```python
from build123d import *

# Parameters (mm, degrees)
F0_W     = 20
F0_H     = 20
F1_DEPTH = 5
F2_R     = 3
F2_R_2   = 1.375
F3_DEPTH = 25
F4_R     = 5
F5_DEPTH = 3.5
F6_R     = 7.5
F7_DEPTH = 1.5


with BuildPart() as f1:
    # F0 (on Top) → F1 (new body)
    with BuildSketch(Plane.XY):
        with Locations((10, 10)):
            Rectangle(F0_W, F0_H)
    extrude(amount=F1_DEPTH)

    # F2 (on face) → F3 (cut)
    with BuildSketch(Plane.XY.offset(5)):
        with Locations((10, 10)):
            Circle(F2_R)
        with Locations((2.5, 17.5)):
            Circle(F2_R_2)
        with Locations((17.5, 17.5)):
            Circle(F2_R_2)
        with Locations((17.5, 2.5)):
            Circle(F2_R_2)
        with Locations((2.5, 2.5)):
            Circle(F2_R_2)
    extrude(amount=-F3_DEPTH, mode=Mode.SUBTRACT)

    # F4 (on face) → F5 (cut)
    with BuildSketch(Plane.XY.offset(5)):
        with Locations((10, 10)):
            Circle(F4_R)
    extrude(amount=-F5_DEPTH, mode=Mode.SUBTRACT)

    # F6 (on face) + F2 (on face) → F7 (cut)
    with BuildSketch(Plane.XY.offset(5)):
        with Locations((10, 10)):
            Circle(F6_R)
    with BuildSketch(Plane.XY.offset(5)):
        with Locations((10, 10)):
            Circle(F2_R)
        with Locations((2.5, 2.5)):
            Circle(F2_R_2)
        with Locations((2.5, 17.5)):
            Circle(F2_R_2)
        with Locations((17.5, 17.5)):
            Circle(F2_R_2)
        with Locations((17.5, 2.5)):
            Circle(F2_R_2)
    extrude(amount=-F7_DEPTH, mode=Mode.SUBTRACT)


solid = f1.part
```
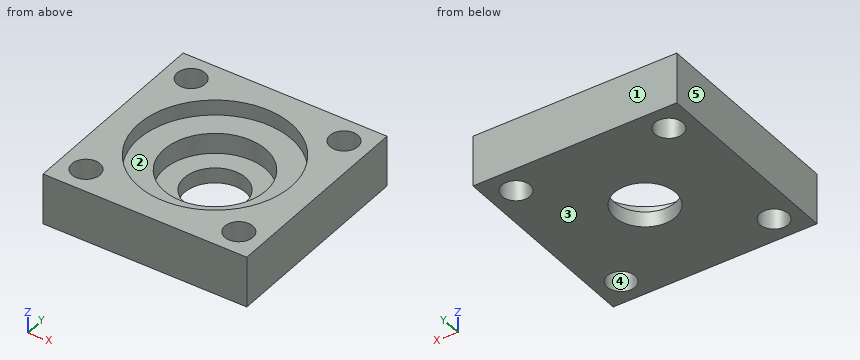
Can you work these out from the model? Positions are in its coordinate system, mm. Face numbers are marked on the shaded views. A direction names the side the tool comes from. Give positions to 0.01 mm unless a question says otherwise; leave off trailing zeros. Order: outer loops, then holes, each group sorted by start corner. A loop starts at its lowest first (then second) coordinate and runs counter-clockwise, first axis right, second up. Notation, with made-up numbers: M 72,47.25 L 103,47.25 A10 cw 103,57.25 Z; hole C 76,65 d3. An arc over 180 degrees is marked long. Write item = value, one per line. Start each with the question number.
Q1. Will these pins go through, and if not, where does the flat tip stop? pin 1 Ø9 at (x, y) = (10, 10) entering from +Z; pin 2 Ø4.5 at (x, y) = (7, 6.5) entering from +Z; pin 3 Ø5 at (x, y) = (10, 10) entering from -Z.
Q2. For the marked faces 1 and 2, which set-ups out of +Z, -Z, +X, -X, +Y, -Y let a thin tool reach every point of the face, with its end or its side?
Q3. I need wall thicknesses on probe 1 along Y at (x, z) = (2.5, 3.15) (3 decimals); probe 2 along Y at (x, z) = (14, 2.1); probe 3 along X at (y, z) = (18.25, 2.6). Which ranges of each line are inside material? Lowest first, please. Write a range as [from, to].
Q4. Suppose I cut it at D-D (y = 16.5). Write out the boundary of the cut face in (x, z), plus the area to 3 significant figures.
Q5. Suppose I cut it at A-A (x = 10). Write out the boundary of the cut face in (y, z).
Q6. Suppose I cut it at C-C (y = 11.25). Write out the boundary of the cut face in (x, z), plus the area to 3 significant figures.
Q7. We'd pull the mould along X, two halves only. Please class the marked faces 3, 4 and 5: pulls with the +X half, pulls with the -X half, needs draft (parallel to the pull), parting line crosses it, or undercut.
Q8. Suppose I cut it at B-B (z = 0.7). Write out the boundary of the cut face in (x, y) (3 decimals).
Check result:
q1.pin_1 = 1.5
q1.pin_2 = 3.5
q1.pin_3 = through
q2.face_1 = +Z, -Z, +X, -X, +Y
q2.face_2 = +Z
q3.probe_1 = [0, 1.125], [3.875, 16.125], [18.875, 20]
q3.probe_2 = [0, 7], [13, 20]
q3.probe_3 = [0, 1.35], [3.65, 16.35], [18.65, 20]
q4.outline = M 0,0 L 1.56,0 L 1.56,5 L 0,5 Z; M 3.44,0 L 16.56,0 L 16.56,5 L 13.74,5 L 13.74,3.5 L 6.26,3.5 L 6.26,5 L 3.44,5 Z; M 18.44,0 L 20,0 L 20,5 L 18.44,5 Z
q4.area = 69.9 mm2
q5.outline = M 0,0 L 7,0 L 7,1.5 L 5,1.5 L 5,3.5 L 2.5,3.5 L 2.5,5 L 0,5 Z; M 13,0 L 20,0 L 20,5 L 17.5,5 L 17.5,3.5 L 15,3.5 L 15,1.5 L 13,1.5 Z
q6.outline = M 0,0 L 7.27,0 L 7.27,1.5 L 5.16,1.5 L 5.16,3.5 L 2.6,3.5 L 2.6,5 L 0,5 Z; M 12.73,0 L 20,0 L 20,5 L 17.4,5 L 17.4,3.5 L 14.84,3.5 L 14.84,1.5 L 12.73,1.5 Z
q6.area = 50.3 mm2
q7.face_3 = needs draft
q7.face_4 = undercut
q7.face_5 = pulls with the -X half
q8.outline = M 0,0 L 20,0 L 20,20 L 0,20 Z; hole C 2.5,2.5 d2.75; hole C 2.5,17.5 d2.75; hole C 10,10 d6; hole C 17.5,2.5 d2.75; hole C 17.5,17.5 d2.75
